Could you check a few things on this model? Use its own coordinates, in mm. A direction names the side the tool comes from. Round coordinates to 2 decimals unless told otherwise and drop trailing zeros. Write each loop counter-clockwise with the first axis right and the second up, starting at its lowest first coordinate (ties: lowest second). Pieces come first, ordered by that corner, then holes. Notation, with made-up numbers: (-7.5, -36.75) -> (22.5, -36.75) arc R20 cw to (22.5, -20.75) -> close; hole circle Ø4 at (79, 26). An arc over 180 degrees is marked (long way). Return JSON: item names as keys, results as strings.
from build123d import *

# Parameters (mm, degrees)
F1_DEPTH = 38.1
F2_W     = 101.6
F2_H     = 47.625
F3_DEPTH = 6.35
F4_W     = 101.6
F4_H     = 47.625
F5_DEPTH = 6.35


# Not quite as in the source:
# - a feature names something its author has since deleted; it is built from what else it names


with BuildPart() as f1:
    # F0 (on Front) → F1 (new body, symmetric)
    with BuildSketch(Plane.XZ):
        Polygon((50.8, 12.2875440849), (50.8, 23.8125), (30.8381908, 23.8125), align=None)
    extrude(amount=F1_DEPTH, both=True)



with BuildPart() as f1b:
    # F0 (on Front) → F1, piece 2 (new body, symmetric)
    with BuildSketch(Plane.XZ):
        Polygon((50.8, -23.8125), (-50.8, 23.8125), (-50.8, -23.8125), align=None)
    extrude(amount=F1_DEPTH, both=True)


with BuildPart() as f1_1:
    add(f1.part)

    add(f1b.part)  # F3 merges F1b
    # F2 (on face) → F3 (join)
    with BuildSketch(Plane(origin=(0, 38.1, 0), x_dir=(-1, 0, 0), z_dir=(0, 1, 0))):
        Rectangle(F2_W, F2_H)
    extrude(amount=-F3_DEPTH)

    # F4 (on face) → F5 (join)
    with BuildSketch(Plane.XZ.offset(38.1)):
        Rectangle(F4_W, F4_H)
    extrude(amount=-F5_DEPTH)


solid = f1_1.part
1) I want a section at B-B, the plane x = 38.5. Please give me the cut outline in (y, z), and give its area (3 significant figures).
Return value:
{"outline": "(-38.1, -23.81) -> (38.1, -23.81) -> (38.1, 23.81) -> (-38.1, 23.81) -> close; hole (-31.75, -18.05) -> (31.75, -18.05) -> (31.75, 19.39) -> (-31.75, 19.39) -> close", "area": "1,250 mm²"}
2) For faces 4 (the face through (12, 31.75, 6)), 5 (the face through (-50.8, -1, 0)), which set-ups out of +Z, -Z, +X, -X, +Y, -Y let a thin tool reach every point of the face, with its end or its side?
Return value:
{"face 4": "none", "face 5": "+Z, -Z, -X, +Y, -Y"}
3) Thinking about a two-plate mould opening in Y: for faces 1 (the face through (0.711, -0.444, -0.333)), 2 (the face through (-1, -38.1, 0)), 3 (the face through (-1, -1, -23.812)), which applies, pulls with the +Y half, pulls with the -Y half, needs draft (parallel to the pull), parting line crosses it, or undercut?
Return value:
{"face 1": "undercut", "face 2": "pulls with the -Y half", "face 3": "needs draft"}
4) I want a section at C-C, the plane y = 7.5. Please give me the cut outline in (x, z), and give its area (3 significant figures).
Return value:
{"outline": "(-50.8, -23.81) -> (50.8, -23.81) -> (-50.8, 23.81) -> close; (30.84, 23.81) -> (50.8, 12.29) -> (50.8, 23.81) -> close", "area": "2,530 mm²"}
5) If I drill on probe 1 along Y at (x, z) = (34, 4); probe 2 along Z at (x, y) = (39.5, 20), over which ranges is the centre line in solid material (lowest first)? Write a range as [from, to].
Return value:
{"probe 1": "[-38.1, -31.75], [31.75, 38.1]", "probe 2": "[-23.81, -18.52], [18.81, 23.81]"}
6) I want a section at A-A, the plane z = 3. Please give me the cut outline in (x, y), and give its area (3 significant figures).
Return value:
{"outline": "(-50.8, -38.1) -> (50.8, -38.1) -> (50.8, -31.75) -> (-6.4, -31.75) -> (-6.4, 31.75) -> (50.8, 31.75) -> (50.8, 38.1) -> (-50.8, 38.1) -> close", "area": "4,110 mm²"}
7) I want a section at D-D, the plane z = 21.5. Please give me the cut outline in (x, y).
Return value:
{"outline": "(-50.8, -38.1) -> (50.8, -38.1) -> (50.8, 38.1) -> (-50.8, 38.1) -> close; hole (-45.87, -31.75) -> (34.84, -31.75) -> (34.84, 31.75) -> (-45.87, 31.75) -> close"}
8) Will these pins go through, and if not, where does the flat tip stop? pin 1 Ø8 at (x, y) = (-36.5, 18.5) entering from +Z; pin 2 Ø5 at (y, z) = (17.5, -3) entering from +X.
Return value:
{"pin 1": "z = 18.98", "pin 2": "x = 11.73"}
